```python
from build123d import *

# Parameters (mm, degrees)
SKETCH1_W           = 45
SKETCH1_H           = 25
BOSS_EXTRUDE1_DEPTH = 12
SKETCH2_R           = 2.5
CUT_EXTRUDE1_DEPTH  = 12
SKETCH3_R           = 2.5
CUT_EXTRUDE2_DEPTH  = 72
SKETCH4_R           = 2.5
CUT_EXTRUDE3_DEPTH  = 72


with BuildPart() as part:
    # Sketch1 → Boss-Extrude1 (new body)
    with BuildSketch(Plane(origin=(0, 0, 0), x_dir=(1, 0, 0), z_dir=(0, 1, 0))):
        Rectangle(SKETCH1_W, SKETCH1_H)
    extrude(amount=BOSS_EXTRUDE1_DEPTH)

    # Sketch2 → Cut-Extrude1 (cut)
    with BuildSketch(Plane(origin=(0, 12, 0), x_dir=(1, 0, 0), z_dir=(0, 1, 0))):
        with Locations((-18, -7.5)):
            Circle(SKETCH2_R)
        with Locations((-18, 7.5)):
            Circle(SKETCH2_R)
        with Locations((18, -7.5)):
            Circle(SKETCH2_R)
        with Locations((18, 7.5)):
            Circle(SKETCH2_R)
    extrude(amount=-CUT_EXTRUDE1_DEPTH, mode=Mode.SUBTRACT)

    # Sketch3 → Cut-Extrude2 (cut)
    with BuildSketch(Plane(origin=(0, 0, -12.5), x_dir=(-1, 0, 0), z_dir=(0, 0, -1))):
        with Locations((0, 6)):
            Circle(SKETCH3_R)
    extrude(amount=-CUT_EXTRUDE2_DEPTH, mode=Mode.SUBTRACT)

    # Sketch4 → Cut-Extrude3 (cut)
    with BuildSketch(Plane(origin=(0, 0, -12.5), x_dir=(-1, 0, 0), z_dir=(0, 0, -1))):
        with Locations((10, 6)):
            Circle(SKETCH4_R)
        with Locations((-10, 6)):
            Circle(SKETCH4_R)
    extrude(amount=-CUT_EXTRUDE3_DEPTH, mode=Mode.SUBTRACT)


solid = part.part
```
Geometry check sheet. Reference: the model listing, model coordinates, mm. Give positions to 0.01 mm unless a question says otherwise; leave off trailing zeros. Loops run counter-clockwise (first coordinate to the right, second up) from the corner with the lowest first, then second, coordinate; pieces in that order, holes last. Notation, with made-up numbers: M 41.25,76.25 L 77.25,76.25 A31 cw 77.25,102.25 Z; hole C 72,-7 d5. An arc over 180 degrees is marked long. Write item = value, one per line. Start each with the question number.
1. Section check C-C, the plane z = -10.5. Enter the section's corners in (x, y), plus the area to 3 significant figures.
2. Thickness scan on probe 1 along Z at (x, y) = (-18, 4.75); probe 2 along Z at (x, y) = (-16.5, 8.5); probe 3 along X at (y, z) = (4.5, -4.5). Record the ranges inside material, lowest first.
3. Section check A-A, the plane z = 7.5. Enter the section's corners in (x, y), plus the area to 3 significant figures.
4. Section check B-B, the plane x = 0. Enter the section's corners in (y, z).
5. Section check D-D, the plane y = 2.25. Enter the section's corners in (x, z).
6. Draft check along Z on faces 1 (the face through (-22.5, 6, 0)), 2 (the face through (-20, 6, -6)), 3 (the face through (-20.5, 6.1, 7.4)), 4 (the face through (0, 3, -12.5)). Enter one of: +Z half, -Z half, draft (parallel to the pull), parting line (faces both ways), or undercut.
Values follow:
q1.outline = M -22.5,0 L 22.5,0 L 22.5,12 L -22.5,12 Z; hole C -10,6 d5; hole C 0,6 d5; hole C 10,6 d5
q1.area = 481 mm^2
q2.probe_1 = -12.5 to -10, -5 to 5, 10 to 12.5
q2.probe_2 = -12.5 to -9.5, -5.5 to 5.5, 9.5 to 12.5
q2.probe_3 = -22.5 to -12, -8 to -2, 2 to 8, 12 to 22.5
q3.outline = M -22.5,0 L -20.5,0 L -20.5,12 L -22.5,12 Z; M -15.5,0 L 15.5,0 L 15.5,12 L -15.5,12 Z; M 20.5,0 L 22.5,0 L 22.5,12 L 20.5,12 Z; hole C -10,6 d5; hole C 0,6 d5; hole C 10,6 d5
q3.area = 361 mm^2
q4.outline = M 0,-12.5 L 3.5,-12.5 L 3.5,12.5 L 0,12.5 Z; M 8.5,-12.5 L 12,-12.5 L 12,12.5 L 8.5,12.5 Z
q5.outline = M -22.5,-12.5 L 22.5,-12.5 L 22.5,12.5 L -22.5,12.5 Z; hole C -18,-7.5 d5; hole C -18,7.5 d5; hole C 18,-7.5 d5; hole C 18,7.5 d5
q6.face_1 = draft
q6.face_2 = undercut
q6.face_3 = undercut
q6.face_4 = -Z half
